Verification items for the finished model (mm, model axes). A direction names the side the tool comes from. Coordinates: 2 decimals unless noted, no trailing zeros. Write each loop counter-clockwise with the first axis right and the second up, starting at its lowest first coordinate (ties: lowest second). Pieces come first, ordered by that corner, then holes. Notation, with made-up numbers: (-33, 23.5) -> (14, 23.5) arc R24 cw to (14, 36.5) -> close; hole circle Ø4 at (-8, 87). An arc over 180 degrees is marked (long way). Answer in a Markdown table with one row per item.
Solid Edge part; units mm, degrees
sketch "Sketch1" plane through (0, 0, 0) normal (0, 0, 1) x (1, 0, 0)
  arc A0 (-26.2419, -8.2226) -> (-6, 26.8375) centre (0, 0) cw
  line L0 (-6, 33.5) -> (-6, 26.8375)
  arc A1 (6, 33.5) -> (-6, 33.5) centre (0, 33.5) ccw
  line L1 (6, 26.8375) -> (6, 33.5)
  arc A2 (6, 26.8375) -> (26.2419, -8.2226) centre (0, 0) cw
  line L2 (32.0119, -11.5538) -> (26.2419, -8.2226)
  arc A3 (26.0119, -21.9462) -> (32.0119, -11.5538) centre (29.0119, -16.75) ccw
  line L3 (20.2419, -18.6149) -> (26.0119, -21.9462)
  arc A4 (20.2419, -18.6149) -> (-20.2419, -18.6149) centre (0, 0) cw
  line L4 (-26.0119, -21.9462) -> (-20.2419, -18.6149)
  arc A5 (-32.0119, -11.5538) -> (-26.0119, -21.9462) centre (-29.0119, -16.75) ccw
  line L5 (-26.2419, -8.2226) -> (-32.0119, -11.5538)
extrude "Protrusion1" add sketch "Sketch1" along normal blind 15
hole "Bohrung_1" at (29.0119, -16.75, 15) direction (0, 0, -1) diameter 6 end through all
hole "Hole1" at (-29.0119, -16.75, 15) direction (0, 0, -1) diameter 6 end through all
hole "Hole2" at (0, 33.5, 15) direction (0, 0, -1) diameter 6 end through all
properties part number "DV5" material "Gelbmessing"
1. Sectioned sample at B-B, the plane y = -16.75. Record the cut outline in (x, z).
Findings below:
| item | result |
|---|---|
| outline | (-35.01, 0) -> (-32.01, 0) -> (-32.01, 15) -> (-35.01, 15) -> close; (-26.01, 0) -> (26.01, 0) -> (26.01, 15) -> (-26.01, 15) -> close; (32.01, 0) -> (35.01, 0) -> (35.01, 15) -> (32.01, 15) -> close |
2. Sectioned sample at C-C, the plane z = 12.5. Record the cut outline in (x, y), and give its area (3 significant figures).
Findings below:
| item | result |
|---|---|
| outline | (-32.01, -11.55) arc R6 ccw to (-26.01, -21.95) -> (-20.24, -18.61) arc R27.5 ccw to (20.24, -18.61) -> (26.01, -21.95) arc R6 ccw to (32.01, -11.55) -> (26.24, -8.22) arc R27.5 ccw to (6, 26.84) -> (6, 33.5) arc R6 ccw to (-6, 33.5) -> (-6, 26.84) arc R27.5 ccw to (-26.24, -8.22) -> close; hole circle Ø6 at (-29.01, -16.75); hole circle Ø6 at (0, 33.5); hole circle Ø6 at (29.01, -16.75) |
| area | 2,680 mm² |
3. Go/stop test with flat-tipped pins: pin 1 (4 mm diameter, centred on x = -22.5, z = 11, fed in from -Y); pin 2 (3.5 mm diameter, centred on y = 30, z = 5, fed in from +X); pin 3 (1 mm diameter, centred on y = 28.5, z = 6, fed in from -X). Record where each tip stops, or that it passes through.
Findings below:
| item | result |
|---|---|
| pin 1 | stops at y = -21.07 |
| pin 2 | stops at x = 6 |
| pin 3 | stops at x = -6 |
4. Sectioned sample at D-D, the plane y = -4.5. Record the cut outline in (x, z), and give its area (3 significant figures).
Findings below:
| item | result |
|---|---|
| outline | (-27.13, 0) -> (27.13, 0) -> (27.13, 15) -> (-27.13, 15) -> close |
| area | 814 mm² |
5. Material ranges on probe 1 along X at (y, z) = (-16.75, 8.25); probe 2 along Y at (x, z) = (0, 10); probe 3 along X at (y, z) = (-17.5, 7.75), recorded low to high. Write a range as from..to.
Findings below:
| item | result |
|---|---|
| probe 1 | x = -35.01..-32.01, -26.01..26.01, 32.01..35.01 |
| probe 2 | y = -27.5..30.5, 36.5..39.5 |
| probe 3 | x = -34.96..-31.92, -26.11..26.11, 31.92..34.96 |
6. Access from +Z, -Z, +X, -X, +Y, -Y to the whole of each face (thin tool, end or side, straight path). Record for faces 1 (the face through (29.167, -9.912, 7.395)), 2 (the face through (-6, 30, 7)), 3 (the face through (-23.167, -20.304, 7.395)), 4 (the face through (6, 30, 7)).
Findings below:
| item | result |
|---|---|
| face 1 | +Z, -Z, +X |
| face 2 | +Z, -Z, -X, +Y |
| face 3 | +Z, -Z, -Y |
| face 4 | +Z, -Z, +X, +Y |
7. Release check for a two-part mould opening along X. For faces 5 (the face through (0, -1, 0)), 6 (the face through (26.083, -16.1, 7.605)), 7 (the face through (-23.973, 13.473, 7.395)), 8 (the face through (23.09, -20.26, 7.4)) record: released by +X, released by -X, zero draft, split by the parting line, or undercut.
Findings below:
| item | result |
|---|---|
| face 5 | zero draft |
| face 6 | undercut |
| face 7 | released by -X |
| face 8 | undercut |
8. Sectioned sample at A-A, the plane x = 0. Record the cut outline in (y, z), and give its area (3 significant figures).
Findings below:
| item | result |
|---|---|
| outline | (-27.5, 0) -> (30.5, 0) -> (30.5, 15) -> (-27.5, 15) -> close; (36.5, 0) -> (39.5, 0) -> (39.5, 15) -> (36.5, 15) -> close |
| area | 915 mm² |
